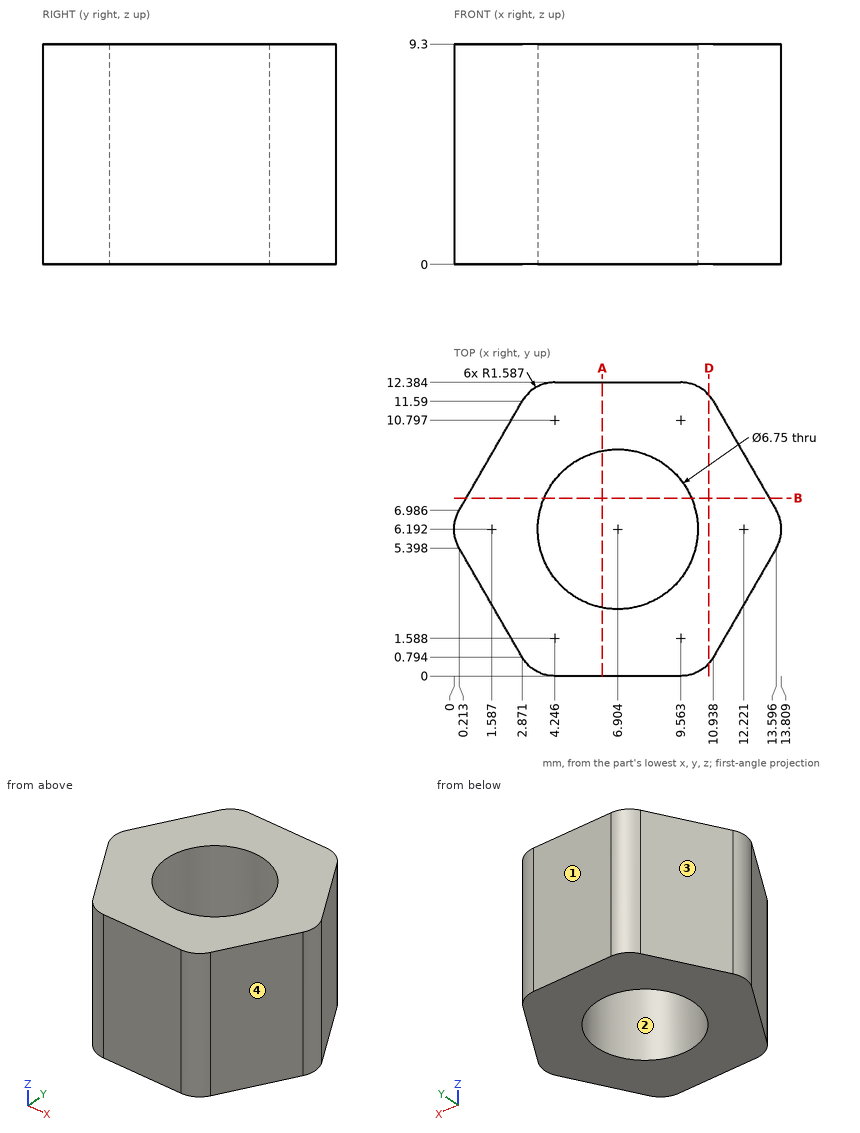
Answer from the drawing. Dimensions are ordinates in mm from the lowest x, y and z of the part. Coordinates: 2 decimals unless noted, no trailing zeros. Loops run counter-clockwise (first coordinate to the right, second up) from the corner with the lowest first, then second, coordinate; pieces in that order, holes last. Notation, with made-up numbers: (44.5, 1) -> (92.5, 1) arc R22 cw to (92.5, 40) -> close; hole circle Ø2 at (41, -7). An arc over 180 degrees is marked (long way). Answer as CSV lines item,"result".
Q1. The part is cut by section B-B on y = 7.5. Write down the section's boundary in (x, z) (1 decimal).
Findings:
outline,"(0.5, 0) -> (3.8, 0) -> (3.8, 9.3) -> (0.5, 9.3) -> close; (10, 0) -> (13.3, 0) -> (13.3, 9.3) -> (10, 9.3) -> close"
Q2. Find the intervals of material crossed by probe 1 along Y at (x, z) = (7, 7) (1 decimal); probe 2 along X at (y, z) = (6.25, 8.25); probe 3 along Y at (x, z) = (5, 8) (1 decimal), in increasing order.
Findings:
probe 1,"y = 0 to 2.8, 9.6 to 12.4"
probe 2,"x = 0 to 3.53, 10.28 to 13.81"
probe 3,"y = 0 to 3.4, 9 to 12.4"
Q3. For a pull along X with two mould halves and no side action, classify the marked faces 1, 2, 3 and 4 as +X half, -X half, draft (parallel to the pull), parting line (faces both ways), or undercut.
Findings:
face 1,"draft"
face 2,"undercut"
face 3,"-X half"
face 4,"+X half"
Q4. The part is cut by section D-D on x = 10.75. Write down the section's boundary in (y, z), and give its area (3 significant figures).
Findings:
outline,"(0.53, 0) -> (11.85, 0) -> (11.85, 9.3) -> (0.53, 9.3) -> close"
area,"105 mm²"
Q5. The part is cut by section A-A on x = 6.25. Write down the section's boundary in (y, z) (1 decimal).
Findings:
outline,"(0, 0) -> (2.9, 0) -> (2.9, 9.3) -> (0, 9.3) -> close; (9.5, 0) -> (12.4, 0) -> (12.4, 9.3) -> (9.5, 9.3) -> close"
Q6. Each of these flat-tipped pins is pushed along its axis until it touches: pin 1 (2 mm diameter, centred on x = 2.5, z = 5, fed in from -Y) (1 decimal); pin 2 (4 mm diameter, centred on y = 8.5, z = 5, fed in from +X). Where does it stop, or does it pass through?
Findings:
pin 1,"stops at y = 0.2"
pin 2,"stops at x = 13.78"
